from build123d import *

# Parameters (mm, degrees)
F1_DEPTH        = 15
F2_W            = 12
F2_H            = 6
F3_DEPTH        = 20
F4_W            = 18
F4_H            = 13
F5_DEPTH        = 13
F6_R            = 3
F7_D            = 3.3
F7_CBORE_D      = 6.5
F7_CBORE_DEPTH  = 6
F9_R            = 2
F10_D           = 1.76
F10_CBORE_D     = 2.2
F10_CBORE_DEPTH = 13


with BuildPart() as f1:
    # F0 (on Front) → F1 (new body)
    with BuildSketch(Plane.XZ):
        Polygon((22, 0), (10, 0), (0, -10), (0, -32), (3, -35), (29, -35), (32, -32), (32, -10), align=None)
    extrude(amount=F1_DEPTH)

    # F2 (on face) → F3 (join)
    with BuildSketch(Plane.XZ.offset(15)):
        with Locations((16, -11)):
            Rectangle(F2_W, F2_H)
    extrude(amount=F3_DEPTH)

    # F4 (on face) → F5 (cut)
    with BuildSketch(Plane(origin=(0, 0, 0), x_dir=(-1, 0, 0), z_dir=(0, 1, 0))):
        with Locations((-16, -11.5)):
            Rectangle(F4_W, F4_H)
    extrude(amount=-F5_DEPTH, mode=Mode.SUBTRACT)

    # F6
    f6_edges = [f1.edges().sort_by_distance(p)[0] for p in [
        (25, -6.5, -5),
        (7, -6.5, -5),
        (25, -6.5, -18),
        (7, -6.5, -18),
    ]]
    fillet(f6_edges, radius=F6_R)

    # F7 (through all)
    with Locations(Plane.XZ.offset(15)):
        with Locations((4, -26.5), (28, -26.5)):
            CounterBoreHole(F7_D / 2, F7_CBORE_D / 2, F7_CBORE_DEPTH)

    # F9
    f9_edges = [f1.edges().sort_by_distance(p)[0] for p in [
        (22, -25, -8),
        (22, -25, -14),
        (10, -25, -8),
        (10, -25, -14),
    ]]
    fillet(f9_edges, radius=F9_R)

    # F10 (through all)
    with Locations(Plane.XZ.offset(35)):
        with Locations((19, -9.7), (16, -9.7), (13, -9.7)):
            CounterBoreHole(F10_D / 2, F10_CBORE_D / 2, F10_CBORE_DEPTH)


solid = f1.part
Design review of the part built by this model. Coordinates are the model's own, in mm. A direction names the side the tool comes from. Coordinates: 2 decimals unless noted, no trailing zeros. Order: outer loops, then holes, each group sorted by start corner. A loop starts at its lowest first (then second) coordinate and runs counter-clockwise, first axis right, second up.
Item 1: The part is to be moulded in two halves that separate along Z. For faces 5 (the cylindrical face through (15.189, -28.591, -8.957)), 6 (the flat face through (16, -6, -18)), 7 (the cylindrical face through (21.43, -25.14, -8.6)), 8 (the cylindrical face through (21.4, -25.14, -13.43)), say which applies: pulls with the +Z half, pulls with the -Z half, needs draft (parallel to the pull), parting line crosses it, or undercut.
Item 2: For faces 1 (the cylindrical face through (7.9, -6.59, -5.86)), 2 (the flat face through (16, -25, -14)), 3 (the flat face through (16, -7, -35)), 4 (the cylindrical face through (17.9, -28.6, -9.7)), list the 3-axis set-ups (+Z, -Z, +X, -X, +Y, -Y) from which the entire face can be reached by the end or side of a thin tool; tool diameter is ignored.
Item 3: For line 1 (X direction, y = -31, z = -9); line 2 (X direction, y = -5.5, z = -11); line 3 (Z direction, x = 13, y = -29.75), list the stretches that pass through material, from the lowest coordinate up.
Item 4: Take a section at B-B, the plane x = 4. Write out the cut boundary in (y, z).
Item 5: Take a section at A-A, the plane z = -26.5. Write out the cut boundary in (x, y), then the cut area to 3 significant figures.
Item 6: Take a section at C-C, the plane y = -18.5. Write out the cut boundary in (x, z).
Item 7: For pin 1 Ø6.5 at (x, y) = (14.5, -28) entering from -Z; pin 2 Ø1.5 at (x, y) = (19.5, -17.5) entering from +Z; pin 3 Ø3 at (x, y) = (7, -24) entering from -Z; pin 4 Ø2 at (y, z) = (-27, -7.5) entering from -X, all flat-tipped, find the tip position at first contact; note any pin that passes through.
Item 8: Take a section at D-D, the plane y = -7. Write out the cut boundary in (x, z).
The answers:
1. face 5: undercut
1. face 6: undercut
1. face 7: pulls with the +Z half
1. face 8: pulls with the -Z half
2. face 1: +Y
2. face 2: -Z, +X, -X, -Y
2. face 3: -Z, +X, -X, +Y, -Y
2. face 4: -Y
3. line 1: x = 10.27 to 12.15, 13.85 to 15.15, 16.85 to 18.15, 19.85 to 21.73
3. line 2: x = 0 to 7, 25 to 32
3. line 3: z = -14 to -10.8, -8.6 to -8
4. outline: (-15, -35) - (0, -35) - (0, -28.15) - (-9, -28.15) - (-9, -29.75) - (-15, -29.75) - close; (-15, -23.25) - (-9, -23.25) - (-9, -24.85) - (0, -24.85) - (0, -6) - (-15, -6) - close
5. outline: (0, -15) - (0.75, -15) - (0.75, -9) - (2.35, -9) - (2.35, 0) - (0, 0) - close; (5.65, -9) - (7.25, -9) - (7.25, -15) - (24.75, -15) - (24.75, -9) - (26.35, -9) - (26.35, 0) - (5.65, 0) - close; (29.65, -9) - (31.25, -9) - (31.25, -15) - (32, -15) - (32, 0) - (29.65, 0) - close
5. area: 343 mm2
6. outline: (10, -12) arc R2 ccw to (12, -14) - (20, -14) arc R2 ccw to (22, -12) - (22, -10) arc R2 ccw to (20, -8) - (12, -8) arc R2 ccw to (10, -10) - close; hole circle Ø1.76 at (13, -9.7); hole circle Ø1.76 at (16, -9.7); hole circle Ø1.76 at (19, -9.7)
7. pin 1: stops at z = -14
7. pin 2: stops at z = -8
7. pin 3: passes through
7. pin 4: stops at x = 10.68
8. outline: (0, -32) - (3, -35) - (29, -35) - (32, -32) - (32, -10) - (22, 0) - (10, 0) - (0, -10) - close; hole circle Ø3.3 at (4, -26.5); hole (7, -15) arc R3 ccw to (10, -18) - (22, -18) arc R3 ccw to (25, -15) - (25, -8) arc R3 ccw to (22, -5) - (10, -5) arc R3 ccw to (7, -8) - close; hole circle Ø3.3 at (28, -26.5)
